Here's how the part is built. I have some questions about the finished solid (model axes, mm). A direction names the side the tool comes from. Round coordinates to 2 decimals unless told otherwise and drop trailing zeros. Order: outer loops, then holes, each group sorted by start corner. A loop starts at its lowest first (then second) coordinate and runs counter-clockwise, first axis right, second up. Notation, with made-up numbers: M -12.5,39 L 37.5,39 A19 ccw 37.5,63 Z; hole C 40,9 d6. An arc over 180 degrees is marked long. Use one line per item in the form item = value. Start each with the question number.
Autodesk Inventor part; units mm, degrees
ref_plane "YZ Plane" through (0, 0, 0) normal (1, 0, 0) x (0, 1, 0)
ref_plane "XZ Plane" through (0, 0, 0) normal (0, 1, 0) x (-1, 0, 0)
ref_plane "XY Plane" through (0, 0, 0) normal (0, 0, 1) x (1, 0, 0)
sketch "Sketch1" plane through (0, 0, 0) normal (0, 0, 1) x (1, 0, 0)
  line L0 (0, 0) -> (58, 0)
  line L1 (58, 0) -> (58, 28)
  line L2 (58, 28) -> (0, 28)
  line L3 (0, 28) -> (0, 0)
  line L4 (22, 12) -> (36, 12)
  line L5 (36, 12) -> (36, 3)
  line L6 (36, 3) -> (22, 3)
  line L7 (22, 3) -> (22, 12)
  line L8 (20, 25) -> (38, 25)
  line L9 (38, 25) -> (38, 15)
  line L10 (38, 15) -> (20, 15)
  line L11 (20, 15) -> (20, 25)
  line L12 (29, 25) -> (29, 3) construction
  point P0 (29, 28)
  point P1 (29, 12)
  point P2 (29, 14)
  point P3 (0, 14)
  dimension "d0" = 14
  dimension "d1" = 9
  dimension "d2" = 28
  dimension "d3" = 58
  dimension "d4" = 18
  dimension "d5" = 10
  dimension "d6" = 3
extrude "Extrusion1" add sketch "Sketch1" along normal blind 25
fillet "Fillet1" radius 5 4 edges at (0, 28, 12.5) (0, 0, 12.5) (58, 0, 12.5) (58, 28, 12.5)
sketch "Sketch2" plane through (0, 0, 25) normal (0, 0, 1) x (1, 0, 0)
  arc A0 (58, 23) -> (53, 28) centre (53, 23) ccw
  line L0 (53, 28) -> (5, 28)
  arc A1 (5, 28) -> (0, 23) centre (5, 23) ccw
  line L1 (0, 23) -> (0, 5)
  arc A2 (0, 5) -> (5, 0) centre (5, 5) ccw
  line L2 (5, 0) -> (53, 0)
  arc A3 (53, 0) -> (58, 5) centre (53, 5) ccw
  line L3 (58, 5) -> (58, 23)
  line L4 (38, 25) -> (38, 15)
  line L5 (38, 15) -> (20, 15)
  line L6 (20, 15) -> (20, 25)
  line L7 (20, 25) -> (38, 25)
  line L8 (36, 12) -> (36, 3)
  line L9 (36, 3) -> (22, 3)
  line L10 (22, 3) -> (22, 12)
  line L11 (22, 12) -> (36, 12)
  line L12 (-8.5, 34) -> (66.5, 34)
  line L13 (66.5, 34) -> (66.5, -6)
  line L14 (66.5, -6) -> (-8.5, -6)
  line L15 (-8.5, -6) -> (-8.5, 34)
  point P0 (29, 34)
  point P1 (29, 28)
  point P2 (0, 14)
  point P3 (-8.5, 14)
  dimension "d11" = 40
  dimension "d12" = 75
extrude "Extrusion2" add sketch "Sketch2" along normal blind 3 contours L3 A3 L2 A2 L1 A1 L0 A0 | L12 L13 L14 L15
chamfer "Chamfer1" distance 10 angle 45 4 edges at (-8.5, 34, 26.5) (-8.5, -6, 26.5) (66.5, 34, 26.5) (66.5, -6, 26.5)
sketch "Sketch3" plane through (0, 0, 25) normal (0, 0, -1) x (-1, 0, 0)
  circle A0 centre (-62.25, 14) radius 2.5
  circle A1 centre (4.25, 14) radius 2.5
  line L0 (-58, 5) -> (-58, 23)
  line L1 (-58, 14) -> (-66.5, 14) construction
  line L2 (-66.5, 24) -> (-66.5, 4) construction
  line L3 (8.5, 4) -> (8.5, 24) construction
  line L4 (0, 23) -> (0, 5) construction
  line L5 (0, 14) -> (8.5, 14) construction
  line L6 (8.5, 24) -> (8.5, 4)
  point P0 (0, 0)
  point P1 (-62.25, 14)
  point P2 (4.25, 14)
  dimension "d18" = 5
  dimension "d19" = 5
extrude "Extrusion3" cut sketch "Sketch3" against normal through all
properties part number "BA28" material "ABS Plastic"
1) On a 3-axis mill with a long thin cutter (end or side, diameter ignored), from which of +Z, -Z, +X, -X, +Y, -Y can I reach the whole of each face in a straight line? I mean faces 4 (the cylindrical face through (56, 1, 13)), 5 (the flat face through (36, 8, 14)), 6 (the cylindrical face through (57, 26, 13)), 7 (the flat face through (29, 28, 12)). Say none if no direction works.
2) If we section it at D-D on x = 62.25: Write out the boundary of the cut face in (y, z).
3) If we section it at A-A on y = 20: Write out the boundary of the cut face in (x, z), then the cut area to 3 significant figures.
4) If we section it at C-C on y = 14: Write out the boundary of the cut face in (x, z).
5) If I drill on line 1 (Y direction, x = 23, z = 10); line 2 (X direction, y = 9.5, z = 14.5); line 3 (X direction, y = 21.5, z = 15), over which ranges is the centre line in solid material (lowest first)?
6) Will these pins go through, and if not, where does the flat tip stop? pin 1 Ø5 at (y, z) = (19, 20.5) entering from +X; pin 2 Ø14.5 at (x, z) = (25, 12.5) entering from -Y; pin 3 Ø4 at (x, z) = (31.5, 18) entering from +Y; pin 4 Ø1 at (x, y) = (25, 27) entering from -Z.
7) If we mould it in two halves opening along Y, with no side actions, what happens to faces 1 (the flat face through (29, 34, 26)), 2 (the flat face through (0, 14, 12)), 3 (the cylindrical face through (59.94, 13.04, 26.48))? For each: +Y half, -Y half, draft (parallel to the pull), parting line (faces both ways), or undercut.
8) If we section it at B-B on z = 14.25: Write out the boundary of the cut face in (x, y), then the cut area to 3 significant figures.
Completed:
q1.face_4 = -Z, +X, -Y
q1.face_5 = +Z, -Z
q1.face_6 = -Z, +X, +Y
q1.face_7 = -Z, +X, -X, +Y
q2.outline = M -0.25,25 L 11.5,25 L 11.5,28 L -0.25,28 Z; M 16.5,25 L 28.25,25 L 28.25,28 L 16.5,28 Z
q3.outline = M -8.5,25 L 0,25 L 0,0 L 20,0 L 20,28 L -8.5,28 Z; M 38,0 L 58,0 L 58,25 L 66.5,25 L 66.5,28 L 38,28 Z
q3.area = 1,170 mm²
q4.outline = M -8.5,25 L -6.75,25 L -6.75,28 L -8.5,28 Z; M -1.75,25 L 0,25 L 0,0 L 58,0 L 58,25 L 59.75,25 L 59.75,28 L -1.75,28 Z; M 64.75,25 L 66.5,25 L 66.5,28 L 64.75,28 Z
q5.line_1 = 0 to 3, 12 to 15, 25 to 28
q5.line_2 = 0 to 22, 36 to 58
q5.line_3 = 0 to 20, 38 to 58
q6.pin_1 = 58
q6.pin_2 = 0
q6.pin_3 = 28
q6.pin_4 = 0
q7.face_1 = +Y half
q7.face_2 = draft
q7.face_3 = undercut
q8.outline = M 0,5 A5 ccw 5,0 L 53,0 A5 ccw 58,5 L 58,23 A5 ccw 53,28 L 5,28 A5 ccw 0,23 Z; hole M 20,15 L 38,15 L 38,25 L 20,25 Z; hole M 22,3 L 36,3 L 36,12 L 22,12 Z
q8.area = 1,300 mm²
